from build123d import *

# Parameters (mm, degrees)
F0_W     = 139.7
F0_H     = 38.1
F1_DEPTH = 25.4
F2_R     = 9.525
F3_DEPTH = 50.801
F4_R     = 5.08
F5_DEPTH = 7.62


with BuildPart() as f1:
    # F0 (on Front) → F1 (new body, symmetric)
    with BuildSketch(Plane.XZ):
        Rectangle(F0_W, F0_H)
    extrude(amount=F1_DEPTH, both=True)

    # F2 (on face) → F3 (cut, through all)
    with BuildSketch(Plane.XZ.offset(25.4)):
        with Locations((-50.8, 0)):
            Circle(F2_R)
        with Locations((50.8, 0)):
            Circle(F2_R)
    extrude(amount=-F3_DEPTH, mode=Mode.SUBTRACT)

    # F4 (on face) → F5 (cut)
    with BuildSketch(Plane.XZ.offset(25.4)):
        with Locations((-10.16, 0)):
            Circle(F4_R)
        with Locations((10.16, 0)):
            Circle(F4_R)
    extrude(amount=-F5_DEPTH, mode=Mode.SUBTRACT)


solid = f1.part
Part model, mm, in its own coordinate system. A direction names the side the tool comes from. Round coordinates to 2 decimals unless told otherwise and drop trailing zeros. Order: outer loops, then holes, each group sorted by start corner. A loop starts at its lowest first (then second) coordinate and runs counter-clockwise, first axis right, second up. Notation, with made-up numbers: (-8.75, 39.25) -> (-0.75, 39.25) arc R35 cw to (-0.75, 77.25) -> close; hole circle Ø10 at (31, 33.5). An arc over 180 degrees is marked (long way). Put each result on its own line as item: value.
Q1. Band-saw the part on A-A (z = 0). Give the cut face in (x, y) (3 decimals).
From the geometry:
outline: (-69.85, -25.4) -> (-60.325, -25.4) -> (-60.325, 25.4) -> (-69.85, 25.4) -> close; (-41.275, -25.4) -> (-15.24, -25.4) -> (-15.24, -17.78) -> (-5.08, -17.78) -> (-5.08, -25.4) -> (5.08, -25.4) -> (5.08, -17.78) -> (15.24, -17.78) -> (15.24, -25.4) -> (41.275, -25.4) -> (41.275, 25.4) -> (-41.275, 25.4) -> close; (60.325, -25.4) -> (69.85, -25.4) -> (69.85, 25.4) -> (60.325, 25.4) -> close
Q2. Wall check: line 1 (Z direction, x = -51, y = 21.5); line 2 (Z direction, x = 10.16, y = -19.5); line 3 (X direction, y = -22, z = 8). Give the ranges that are in metal, low to high. Write a range as [from, to].
From the geometry:
line 1: z = [-19.05, -9.52], [9.52, 19.05]
line 2: z = [-19.05, -5.08], [5.08, 19.05]
line 3: x = [-69.85, -55.97], [-45.63, 45.63], [55.97, 69.85]
Q3. Band-saw the part on D-D (x = -10.16). Give the cut face in (y, z).
From the geometry:
outline: (-25.4, -19.05) -> (25.4, -19.05) -> (25.4, 19.05) -> (-25.4, 19.05) -> (-25.4, 5.08) -> (-17.78, 5.08) -> (-17.78, -5.08) -> (-25.4, -5.08) -> close
Q4. Pull direction X, two halves, no side cores. Call faces 1 (the face through (-69.85, 0, 0)), 2 (the face through (-1, 0, 19.05)), 3 (the face through (69.85, 0, 0)), 4 (the face through (10, -17.78, 0)): pulls with the +X half, pulls with the -X half, needs draft (parallel to the pull), parting line crosses it, or undercut.
From the geometry:
face 1: pulls with the -X half
face 2: needs draft
face 3: pulls with the +X half
face 4: undercut
Q5. Band-saw the part on C-C (y = 11). Give the cut face in (x, z) (3 decimals), and give its area (3 significant figures).
From the geometry:
outline: (-69.85, -19.05) -> (69.85, -19.05) -> (69.85, 19.05) -> (-69.85, 19.05) -> close; hole circle Ø19.05 at (-50.8, 0); hole circle Ø19.05 at (50.8, 0)
area: 4,750 mm2
Q6. Pin check, flat tip, straight feed: pin 1 Ø11.5 at (x, z) = (-50.8, 0) entering from -Y. Stop position of the tip, or through.
From the geometry:
pin 1: passes through
Q7. Tool access for faces 5 (the face through (-1, 25.4, 0)), 6 (the face through (-14.19, -21.64, -3.09)): list every direction of +Z, -Z, +X, -X, +Y, -Y with a clear straight run to the whole face (end or side of a thin tool).
From the geometry:
face 5: +Z, -Z, +X, -X, +Y
face 6: -Y
Q8. Band-saw the part on B-B (x = 50.8). Give the cut face in (y, z) (3 decimals).
From the geometry:
outline: (-25.4, -19.05) -> (25.4, -19.05) -> (25.4, -9.525) -> (-25.4, -9.525) -> close; (-25.4, 9.525) -> (25.4, 9.525) -> (25.4, 19.05) -> (-25.4, 19.05) -> close
